Check sheet for the drawn part. Datum: minimum x, y, z corner. Units: mm. Give positions to 0.01 mm unless a question says otherwise; leave off trailing zeros. Order: outer loops, then holes, each group sorted by start corner. A loop starts at its lowest first (then second) coordinate and runs counter-clockwise, first axis right, second up.
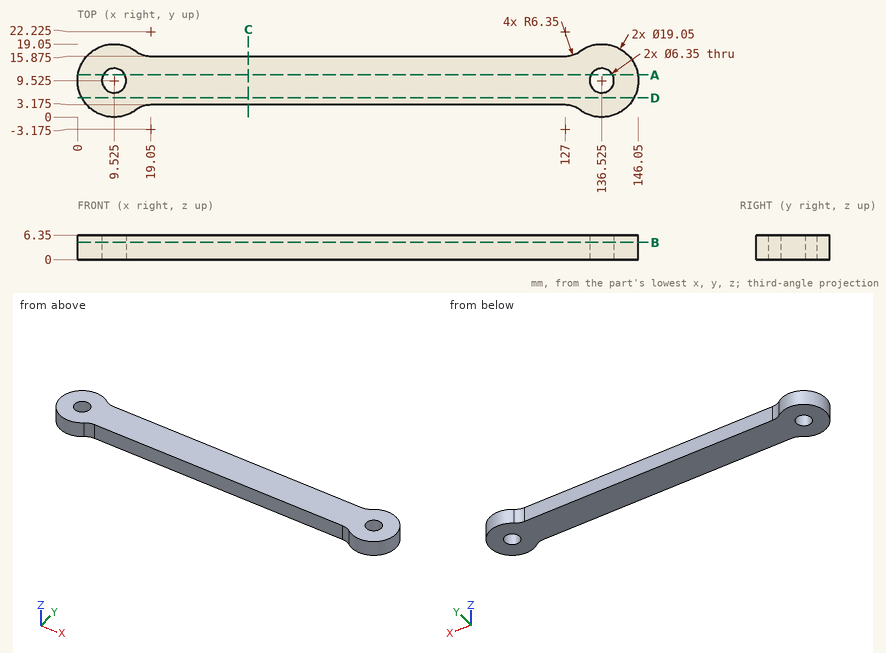
Q1. Go/stop test with flat-tipped pins: P1, Ø5.5, axis at x = 136.525, y = 9.525, coming from the -Z side; P2, Ø3, axis at x = 59, z = 3, coming from the -Y side (3 decimals); P3, Ø1.5, axis at x = 75, z = 4, coming from the +Y side (3 decimals); P4, Ø1, axis at y = 5.5, z = 3.5, coming from the -X side. Record where each tip stops, or that it passes through.
Q2. Sectioned sample at B-B, the plane z = 4.5. Record the cut outline in (x, y) (3 decimals).
Q3. Sectioned sample at C-C, the plane x = 44.5. Record the cut outline in (y, z) (3 decimals).
Q4. Sectioned sample at A-A, the plane y = 11. Record the cut outline in (x, z).
Q5. Sectioned sample at D-D, the plane y = 5. Record the cut outline in (x, z), plus the area to 3 significant figures.
Q6. Material ranges on line 1 (X direction, y = 9.75, z = 4.5); line 2 (X direction, y = 11.25, z = 5); line 3 (Y direction, x = 103.5, z = 5.25) (3 decimals), recorded low to high.
Filled in:
1. P1: passes through
1. P2: stops at y = 3.175
1. P3: stops at y = 15.875
1. P4: stops at x = 0.68
2. outline: (15.24, 1.905) arc R6.35 cw to (19.05, 3.175) - (127, 3.175) arc R6.35 cw to (130.81, 1.905) arc R9.525 ccw (long way) to (130.81, 17.145) arc R6.35 cw to (127, 15.875) - (19.05, 15.875) arc R6.35 cw to (15.24, 17.145) arc R9.525 ccw (long way) to start; hole circle Ø6.35 at (9.525, 9.525); hole circle Ø6.35 at (136.525, 9.525)
3. outline: (3.175, 0) - (15.875, 0) - (15.875, 6.35) - (3.175, 6.35) - close
4. outline: (0.11, 0) - (6.71, 0) - (6.71, 6.35) - (0.11, 6.35) - close; (12.34, 0) - (133.71, 0) - (133.71, 6.35) - (12.34, 6.35) - close; (139.34, 0) - (145.94, 0) - (145.94, 6.35) - (139.34, 6.35) - close
5. outline: (1.14, 0) - (144.91, 0) - (144.91, 6.35) - (1.14, 6.35) - close
5. area: 913 mm2
6. line 1: x = 0 to 6.36, 12.69 to 133.36, 139.69 to 146.05
6. line 2: x = 0.16 to 6.86, 12.19 to 133.86, 139.19 to 145.89
6. line 3: y = 3.175 to 15.875
